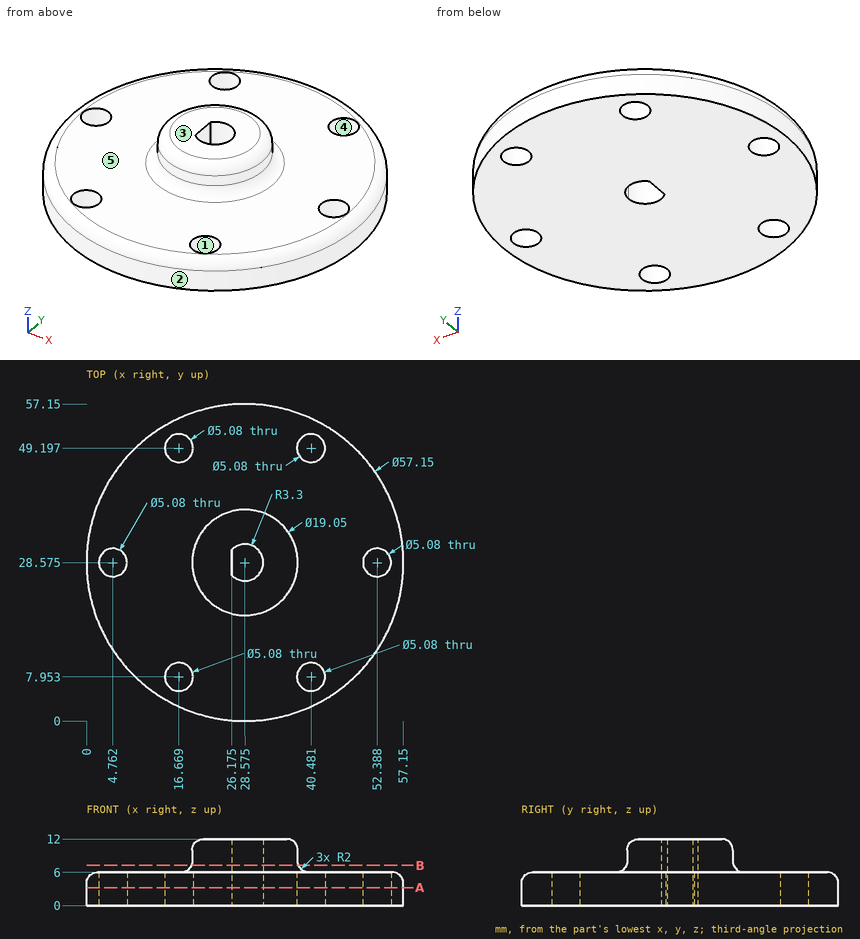
Geometry check sheet. Reference: drawing and pictorial views, mm from the part's lowest x, y, z. A direction names the side the tool comes from. Round coordinates to 2 decimals unless told otherwise and drop trailing zeros. Write each loop counter-clockwise with the first axis right and the second up, starting at its lowest first coordinate (ties: lowest second). Pieces come first, ordered by that corner, then holes.
1. Draft check along X on the marked faces 1, 2 and 3. Enter one of: +X half, -X half, draft (parallel to the pull), parting line (faces both ways), or undercut.
2. Access from +Z, -Z, +X, -X, +Y, -Y to the whole of each face (thin tool, end or side, straight path). Record for the marked faces 4 and 5.
3. Scan lines: L1, parallel to X at y = 8.5, z = 0.75; L2, parallel to Z at x = 18.5, y = 52.5; L3, parallel to X at y = 9.5, z = 5 (1 decimal). Record each from-to range of solid material in increasing order.
4. Section check A-A on z = 3.25. State how many separate pieces and enclosed holes the cut face has, plus the area to 3 significant figures.
5. Section check B-B on z = 7.25. Enter the section's corners in (x, y) (1 decimal), plus the area to 3 significant figures.
6. Gauge pin test, flat ends, axial feed: P1, Ø4.5, axis at x = 16.67, y = 7.95, coming from the +Z side; P2, Ø1.5, axis at x = 32.5, y = 47.5, coming from the +Z side; P3, Ø2, axis at y = 47.5, z = 4, coming from the -X side; P4, Ø1, axis at y = 23.5, z = 8.5, coming from the -X side. Record the tip position at first contact, or that the pin passes through.
Answer:
1. face 1: undercut
1. face 2: parting line
1. face 3: draft
2. face 4: +Z, -Z
2. face 5: +Z
3. L1: x = 8.24 to 14.19, 19.15 to 38, 42.96 to 48.91
3. L2: z = 0 to 6
3. L3: x = 7.7 to 14.7, 18.7 to 38.5, 42.5 to 49.5
4. separate pieces: 1
4. enclosed holes: 7
4. area: 2,410 mm2
5. outline: circle Ø19.3 at (28.6, 28.6); hole (26.2, 26.3) arc R3.3 ccw (long way) to (26.2, 30.8) - close
5. area: 262 mm2
6. P1: passes through
6. P2: stops at z = 6
6. P3: stops at x = 6.32
6. P4: stops at x = 20.22
